Part print with two shaded views. Sizes in mm from the minimum x, y, z corner. Coordinates: 2 decimals unless noted, no trailing zeros. Write each loop counter-clockwise with the first axis right and the second up, starting at its lowest first coordinate (ties: lowest second). Pieces come first, ordered by that corner, then holes. Notation, with made-up numbers: M 37,72.5 L 72,72.5 A27 cw 72,98.5 Z; hole C -28,-29 d9. An arc over 180 degrees is marked long. Answer in a Markdown table with one row per item. Add a question column.
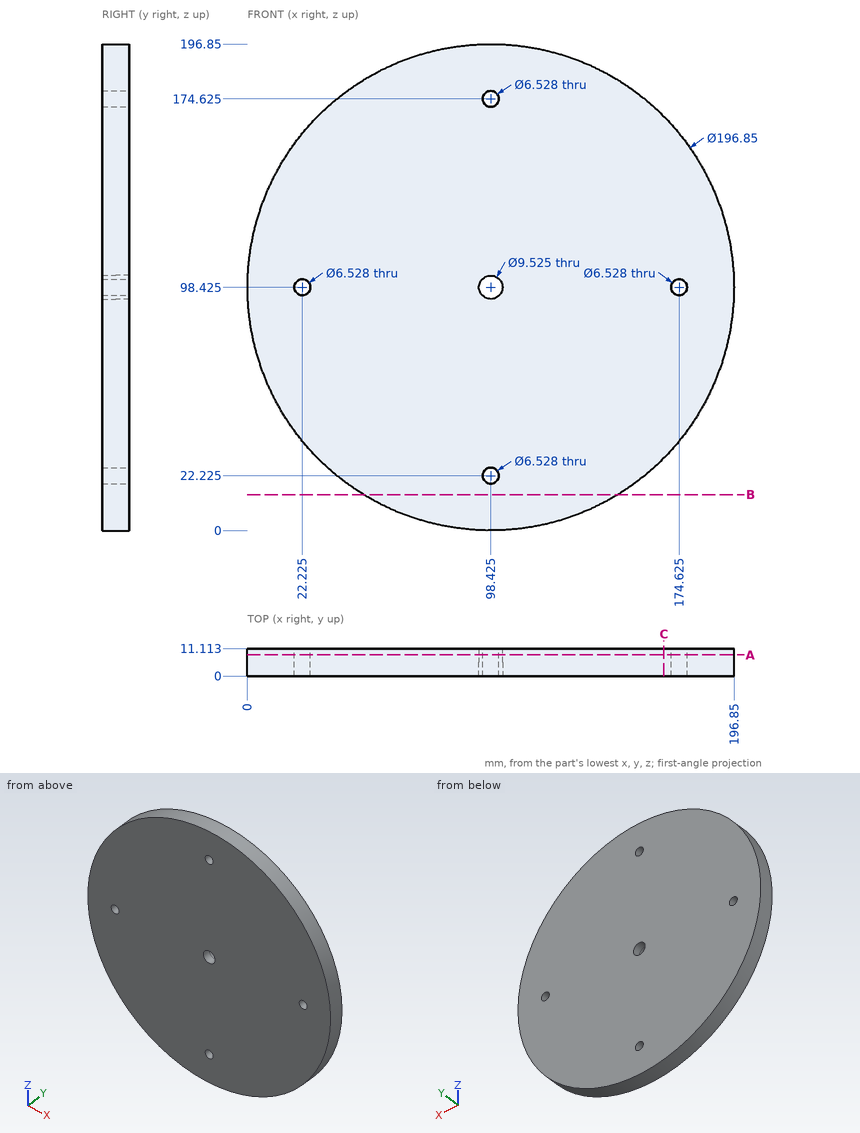
1) Drill centre lines: probe 1 along X at (y, z) = (9.75, 45); probe 2 along Z at (x, y) = (122, 4.25) (1 decimal); probe 3 along X at (y, z) = (2.5, 146.5). Where is each one in solid material? Low to high.
2) Slice it at C-C (x = 168.5). Give the cut face in (y, z).
3) Slice it at B-B (z = 14.5). Give the cut face in (x, y) (1 decimal), then the cut area to 3 significant figures.
4) Flat gauge pins, fed straight in: pin 1 Ø5.5 at (x, z) = (98.425, 98.425) entering from +Y; pin 2 Ø2 at (y, z) = (7.5, 31) entering from -X (1 decimal); pin 3 Ø4 at (y, z) = (8.5, 165.5) entering from +X; pin 4 Ø7.5 at (x, z) = (98.425, 174.625) entering from +Y. Where does each tip first touch, or does it go through?
5) Slice it at A-A (y = 8.5). Count the separate pieces of the cut face and the enclosed holes in it, then the cut area to 3 significant figures.
Ans:
| question | item | result |
|---|---|---|
| 1 | probe 1 | x = 15.76 to 181.09 |
| 1 | probe 2 | z = 2.9 to 194 |
| 1 | probe 3 | x = 12.54 to 184.31 |
| 2 | outline | M 0,29.31 L 11.11,29.31 L 11.11,167.54 L 0,167.54 Z |
| 3 | outline | M 47,0 L 149.8,0 L 149.8,11.1 L 47,11.1 Z |
| 3 | area | 1,140 mm2 |
| 4 | pin 1 | passes through |
| 4 | pin 2 | stops at x = 25.8 |
| 4 | pin 3 | stops at x = 172.27 |
| 4 | pin 4 | stops at y = 11.11 |
| 5 | separate pieces | 1 |
| 5 | enclosed holes | 5 |
| 5 | area | 30,200 mm2 |
